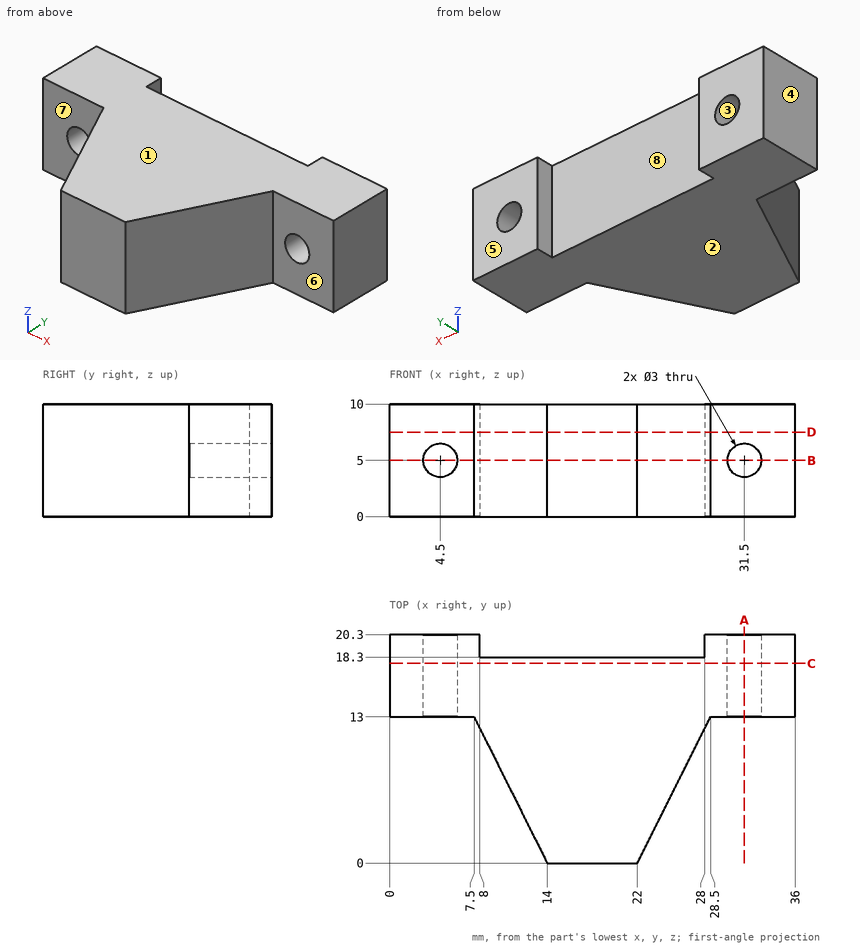
Here's the drawing with two shaded views (mm, measured from the low corner). I have some questions. A direction names the side the tool comes from. Coordinates: 2 decimals unless noted, no trailing zeros. Write each loop counter-clockwise with the first axis right and the second up, starting at its lowest first coordinate (ties: lowest second). Pieces come first, ordered by that corner, then holes. Notation, with made-up numbers: (78.5, 65.5) - (116.5, 65.5) arc R21 ccw to (116.5, 89.5) - close; hole circle Ø3 at (-6.75, 53). An arc over 180 degrees is marked (long way). Return JSON: item names as keys, results as strings.
Q1. I'm going to push flat-ended pins straight in: pin 1 Ø3 at (x, z) = (18, 4) entering from +Y; pin 2 Ø3 at (x, z) = (9.5, 7) entering from -Y; pin 3 Ø1.6 at (y, z) = (19.5, 3.5) entering from -X; pin 4 Ø5 at (x, z) = (26.5, 6.5) entering from -Y. Where does each tip first touch, or does it pass through?
Computed values:
{"pin 1": "stops at y = 18.3", "pin 2": "stops at y = 6", "pin 3": "stops at x = 0", "pin 4": "stops at y = 4"}
Q2. Thinking about a two-plate mould opening in Z: for the marked faces 1, 2, 3 and 4, which applies, +Z half, -Z half, draft (parallel to the pull), parting line (faces both ways), or undercut?
Computed values:
{"face 1": "+Z half", "face 2": "-Z half", "face 3": "undercut", "face 4": "draft"}
Q3. If we section it at D-D (z = 7.5): Please give me the cut outline in (x, y), then the cut area to 3 significant figures.
Computed values:
{"outline": "(0, 13) - (7.5, 13) - (14, 0) - (22, 0) - (28.5, 13) - (36, 13) - (36, 20.3) - (28, 20.3) - (28, 18.3) - (8, 18.3) - (8, 20.3) - (0, 20.3) - close", "area": "411 mm2"}
Q4. Please list where these lines run through material, in increasing order: L1, parallel to Z at x = 4.5, y = 17.25; L2, parallel to X at y = 15.5, z = 5; L3, parallel to X at y = 15.75, z = 3.75. Write a range as from..to.
Computed values:
{"L1": "z = 0..3.5, 6.5..10", "L2": "x = 0..3, 6..30, 33..36", "L3": "x = 0..3.67, 5.33..30.67, 32.33..36"}
Q5. If we section it at B-B (z = 5): Please give me the cut outline in (x, y).
Computed values:
{"outline": "(0, 13) - (3, 13) - (3, 20.3) - (0, 20.3) - close; (6, 13) - (7.5, 13) - (14, 0) - (22, 0) - (28.5, 13) - (30, 13) - (30, 20.3) - (28, 20.3) - (28, 18.3) - (8, 18.3) - (8, 20.3) - (6, 20.3) - close; (33, 13) - (36, 13) - (36, 20.3) - (33, 20.3) - close"}
Q6. If we section it at C-C (y = 17.75): Please give me the cut outline in (x, z).
Computed values:
{"outline": "(0, 0) - (36, 0) - (36, 10) - (0, 10) - close; hole circle Ø3 at (4.5, 5); hole circle Ø3 at (31.5, 5)"}
Q7. On a 3-axis mill with a long thin cutter (end or side, diameter ignored), from which of +Z, -Z, +X, -X, +Y, -Y can I reach the whole of each face in a straight line? I mean the marked faces 5, 6, 7 and 8. Say none if no direction works.
Computed values:
{"face 5": "+Z, -Z, +X, -X, +Y", "face 6": "+Z, -Z, +X, -Y", "face 7": "+Z, -Z, -X, -Y", "face 8": "+Z, -Z, +Y"}
Q8. If we section it at A-A (x = 31.5): Please give me the cut outline in (y, z).
Computed values:
{"outline": "(13, 0) - (20.3, 0) - (20.3, 3.5) - (13, 3.5) - close; (13, 6.5) - (20.3, 6.5) - (20.3, 10) - (13, 10) - close"}
